Work out the finished part from the listing and answer in its coordinate system (mm). Face numbers are marked on the shaded views. A direction names the side the tool comes from. Round coordinates to 2 decimals unless told otherwise and drop trailing zeros. Loops run counter-clockwise (first coordinate to the right, second up) from the corner with the lowest first, then second, coordinate; pieces in that order, holes last. Notation, with made-up numbers: (1.5, -13) - (20.5, -13) arc R29 ccw to (20.5, 16) - close; hole circle Ø2 at (57.25, 19.5). An arc over 180 degrees is marked (long way). Answer as CSV lines item,"result". Start each with the question number.
Q1. Section B-B on z = 12.5 is taken. Write down the section's boundary in (x, y).
Q2. Each of these flat-tipped pins is pushed along its axis until it touches: pin 1 Ø8 at (y, z) = (16, 10) entering from +X; pin 2 Ø11 at (x, y) = (8.5, 50) entering from -Z; pin 3 Ø19.5 at (x, z) = (51.5, 23) entering from +Y. Where does it stop, or does it pass through?
Q3. For the marked faces 1 and 2, determine the directions among +Z, -Z, +X, -X, +Y, -Y from which every point of the face is accessible in a straight line to the end or side of a thin tool.
Q4. Straight lines are drawn through the part: L1, parallel to X at y = 27, z = 26.5; L2, parallel to Z at x = 83.5, y = 16.5. For each, find the intervals that lie inside material, in ascending order. Write a range as [from, to].
Q5. Section A-A on x = 52 is taken. Write down the section's boundary in (y, z), then the cut area to 3 significant figures.
Q6. The mould has two halves that part along Z. Classify the marked faces 3, 4 and 5: +Z half, -Z half, draft (parallel to the pull), parting line (faces both ways), or undercut.
```python
from build123d import *

# Parameters (mm, degrees)
SCHIZZO1_W                   = 5
SCHIZZO1_H                   = 70
ESTRUSIONE_ESTRUSIONE1_DEPTH = 70
ESTRUSIONE_ESTRUSIONE2_START = -35
ESTRUSIONE_ESTRUSIONE2_DEPTH = 5
SCHIZZO3_R                   = 2.5
ESTRUSIONE_ESTRUSIONE3_DEPTH = 5
SCHIZZO4_W                   = 130
SCHIZZO4_H                   = 70
ESTRUSIONE_ESTRUSIONE4_DEPTH = 5
SCHIZZO5_R                   = 1.25
TAGLIO_ESTRUSIONE1_DEPTH     = 46
ESTRUSIONE_ESTRUSIONE5_DEPTH = 3
RACCORDO1_R                  = 5
RACCORDO2_R                  = 5
RACCORDO3_R                  = 2
RACCORDO4_R                  = 2


with BuildPart() as part:
    # Schizzo1 → Estrusione-Estrusione1 (new body)
    with BuildSketch(Plane.XY):
        with Locations((-2.5, 35)):
            Rectangle(SCHIZZO1_W, SCHIZZO1_H)
    extrude(amount=ESTRUSIONE_ESTRUSIONE1_DEPTH)

    # Schizzo2 → Estrusione-Estrusione2 (add)
    with BuildSketch(Plane.XY.offset(70).offset(ESTRUSIONE_ESTRUSIONE2_START)):
        with BuildLine():
            Line((0, 50), (0, 45))
            Line((0, 45), (7.531619243, 45))
            ThreePointArc((7.531619243, 45), (12.531619243, 50), (7.531619243, 55))
            Line((7.531619243, 55), (0, 55))
            Line((0, 55), (0, 50))
        make_face()
        with BuildLine():
            Line((0, 20), (0, 15))
            Line((0, 15), (7.531619243, 15))
            ThreePointArc((7.531619243, 15), (12.531619243, 20), (7.531619243, 25))
            Line((7.531619243, 25), (0, 25))
            Line((0, 25), (0, 20))
        make_face()
    extrude(amount=-ESTRUSIONE_ESTRUSIONE2_DEPTH)

    # Schizzo3 → Estrusione-Estrusione3 (add)
    with BuildSketch(Plane(origin=(0, 0, 30), x_dir=(-1, 0, 0), z_dir=(0, 0, -1))):
        with Locations((-7.547600082, 50.061310314)):
            Circle(SCHIZZO3_R)
        with Locations((-7.547600082, 19.939772921)):
            Circle(SCHIZZO3_R)
    extrude(amount=ESTRUSIONE_ESTRUSIONE3_DEPTH)

    # Schizzo4 → Estrusione-Estrusione4 (add)
    with BuildSketch(Plane.XZ):
        with Locations((60, 35)):
            Rectangle(SCHIZZO4_W, SCHIZZO4_H)
    extrude(amount=ESTRUSIONE_ESTRUSIONE4_DEPTH)

    # Schizzo5 → Taglio-Estrusione1 (cut, through all)
    with BuildSketch(Plane(origin=(0, 0, 25), x_dir=(-1, 0, 0), z_dir=(0, 0, -1))):
        with Locations((-7.547600082, 50.061310314)):
            Circle(SCHIZZO5_R)
        with Locations((-7.547600082, 19.939772921)):
            Circle(SCHIZZO5_R)
    extrude(amount=-TAGLIO_ESTRUSIONE1_DEPTH, mode=Mode.SUBTRACT)

    # Schizzo6 → Estrusione-Estrusione5 (add)
    with BuildSketch(Plane.XY.offset(70)):
        Polygon((125, 0), (0, 0), (0, 70), (-5, 70), (-5, -5), (125, -5), align=None)
        Polygon((0, 70), (125, 0), (0, 0), align=None)
    extrude(amount=ESTRUSIONE_ESTRUSIONE5_DEPTH)

    # Raccordo1
    raccordo1_edges = [part.edges().sort_by_distance(p)[0] for p in [
        (0, 35, 70),
        (62.5, 0, 70),
        (0, 0, 35),
    ]]
    fillet(raccordo1_edges, radius=RACCORDO1_R)

    # Raccordo2
    raccordo2_edges = [part.edges().sort_by_distance(p)[0] for p in [
        (0, 50, 35),
        (0, 20, 35),
    ]]
    fillet(raccordo2_edges, radius=RACCORDO2_R)

    # Raccordo3
    raccordo3_edges = [part.edges().sort_by_distance(p)[0] for p in [
        (0, 50, 30),
        (0, 20, 30),
    ]]
    fillet(raccordo3_edges, radius=RACCORDO3_R)

    # Raccordo4
    raccordo4_edges = [part.edges().sort_by_distance(p)[0] for p in [
        (0, 25, 32.5),
        (0, 15, 32.5),
        (0, 45, 32.5),
        (0, 55, 32.5),
    ]]
    fillet(raccordo4_edges, radius=RACCORDO4_R)


solid = part.part
```
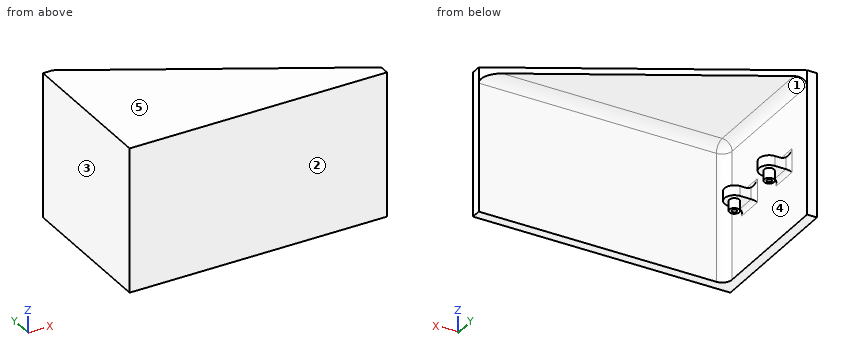
Findings:
1,outline,"(-5, -5) - (125, -5) - (125, 0) - (5, 0) arc R5 cw to (0, 5) - (0, 70) - (-5, 70) - close"
2,pin 1,"stops at x = 0"
2,pin 2,"stops at z = 25"
2,pin 3,"stops at y = 0"
3,face 1,"+X, +Y"
3,face 2,"+Z, -Z, +X, -X, -Y"
4,L1,"x = [-5, 0]"
4,L2,"z = [70, 73]"
5,outline,"(-5, 0) - (0, 0) - (0, 65) arc R5 cw to (5, 70) - (40.88, 70) - (40.88, 73) - (-5, 73) - close"
5,area,"493 mm^2"
6,face 3,"draft"
6,face 4,"undercut"
6,face 5,"+Z half"
